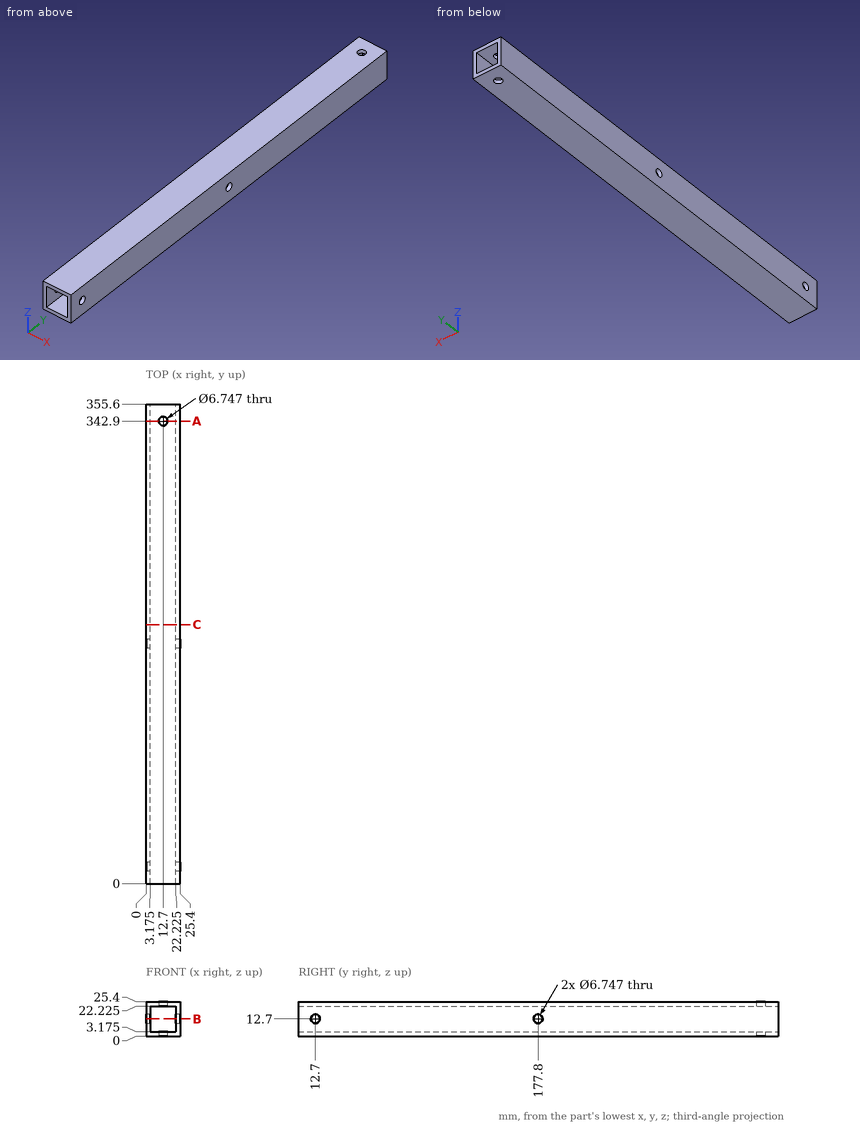
Can you work these out from the drawing? Everything is in mm from the part's minimum corner. Give positions to 0.01 mm unless a question says otherwise; leave off trailing zeros. Order: outer loops, then holes, each group sorted by start corner. A loop starts at its lowest first (then second) coordinate and runs counter-clockwise, first axis right, second up. Notation, with made-up numbers: (37, 34) -> (77, 34) arc R26 cw to (77, 67) -> close; hole circle Ø4 at (89, 61.5). An arc over 180 degrees is marked (long way). Return JSON: item names as keys, results as strings.
1. Imagine slicing it at C-C on y = 192. List the corners of the cut face in (x, z) for me (3 decimals), then the cut area to 3 significant figures.
Answer list:
{"outline": "(0, 0) -> (25.4, 0) -> (25.4, 25.4) -> (0, 25.4) -> close; hole (3.175, 3.175) -> (22.225, 3.175) -> (22.225, 22.225) -> (3.175, 22.225) -> close", "area": "282 mm2"}
2. I need wall thicknesses on line 1 (Y direction, x = 1.1, z = 12.7); line 2 (Z direction, x = 12.5, y = 215) (3 decimals); line 3 (Y direction, x = 12.7, z = 0.75). Which ranges of each line are inside material? Lowest first, please. Write a range as from..to.
Answer list:
{"line 1": "y = 0..9.33, 16.07..174.43, 181.17..355.6", "line 2": "z = 0..3.175, 22.225..25.4", "line 3": "y = 0..339.53, 346.27..355.6"}
3. Imagine slicing it at A-A on y = 342.9. List the corners of the cut face in (x, z) for me (1 decimal), then the cut area to 3 significant figures.
Answer list:
{"outline": "(0, 0) -> (9.3, 0) -> (9.3, 3.2) -> (3.2, 3.2) -> (3.2, 22.2) -> (9.3, 22.2) -> (9.3, 25.4) -> (0, 25.4) -> close; (16.1, 0) -> (25.4, 0) -> (25.4, 25.4) -> (16.1, 25.4) -> (16.1, 22.2) -> (22.2, 22.2) -> (22.2, 3.2) -> (16.1, 3.2) -> close", "area": "239 mm2"}
4. For pin 1 Ø4 at (y, z) = (12.7, 12.7) entering from +X, with a flat end and sliding along its axis, tell me the tip position at first contact or that it passes through.
Answer list:
{"pin 1": "passes through"}
5. Imagine slicing it at B-B on z = 12.7. List the corners of the cut face in (x, y) for me (1 decimal).
Answer list:
{"outline": "(0, 0) -> (3.2, 0) -> (3.2, 9.3) -> (0, 9.3) -> close; (0, 16.1) -> (3.2, 16.1) -> (3.2, 174.4) -> (0, 174.4) -> close; (0, 181.2) -> (3.2, 181.2) -> (3.2, 355.6) -> (0, 355.6) -> close; (22.2, 0) -> (25.4, 0) -> (25.4, 9.3) -> (22.2, 9.3) -> close; (22.2, 16.1) -> (25.4, 16.1) -> (25.4, 174.4) -> (22.2, 174.4) -> close; (22.2, 181.2) -> (25.4, 181.2) -> (25.4, 355.6) -> (22.2, 355.6) -> close"}
